Source: CAD feature listing. Evaluate the final solid. Frame: model axes, mm. Face numbers are marked on the shaded views. A direction names the side the tool comes from. Coordinates: 2 decimals unless noted, no trailing zeros. Order: outer loops, then holes, each group sorted by start corner. A loop starts at its lowest first (then second) coordinate and runs counter-clockwise, first axis right, second up.
Item 1: Contact query for flat-ended pins moving along their axis: P1, Ø0.8, axis at x = 2, z = 0, coming from the +Y side; P2, Ø2, axis at y = 1, z = -26, coming from the +X side; P3, Ø1.5, axis at y = 5, z = 0, coming from the -X side. Output: stop coordinate, or through.
Item 2: Section C-C on y = 5. Return the cut outline in (x, z), then the cut area to 3 significant figures.
Item 3: Reachability of the marked faces 1 and 2 from +Z, -Z, +X, -X, +Y, -Y: full face, straight path, thin tool, end or side. Return the list, or none.
Item 4: Section D-D on x = -3.25. Return the cut outline in (y, z), then the cut area to 3 significant figures.
Item 5: Section A-A on z = 0. Return the cut outline in (x, y).
Item 6: Ray query, line 1 (X direction, y = 6.85, z = 0); line 2 (Y direction, x = 1.75, z = -10). Return the intervals inside material, ascending.
Item 7: Section B-B on x = 1. Return the cut outline in (y, z).
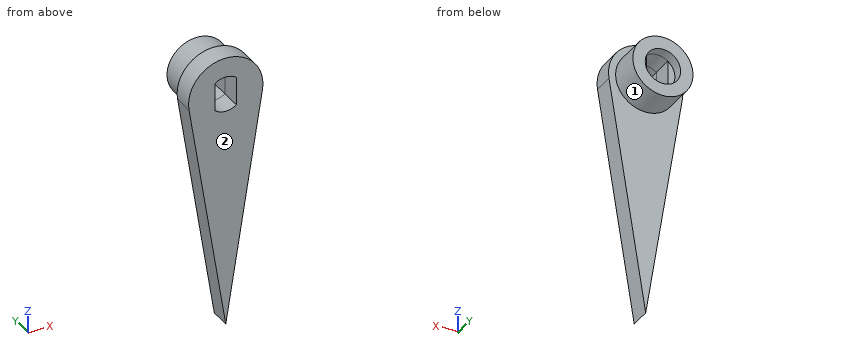
from build123d import *

# Parameters (mm, degrees)
SKETCH5_R           = 4.25
BOSS_EXTRUDE3_DEPTH = 7.5
SKETCH7_R           = 2.5
CUT_EXTRUDE2_DEPTH  = 1.5
CUT_EXTRUDE3_DEPTH  = 6
SKETCH9_R           = 5.25
BOSS_EXTRUDE4_DEPTH = 3


with BuildPart() as part:
    # Sketch5 → Boss-Extrude3 (new body)
    with BuildSketch(Plane(origin=(0, 0, 0), x_dir=(1, 0, 0), z_dir=(0, 1, 0))):
        Circle(SKETCH5_R)
    extrude(amount=BOSS_EXTRUDE3_DEPTH)

    # Sketch7 → Cut-Extrude2 (cut)
    with BuildSketch(Plane(origin=(0, 7.5, 0), x_dir=(1, 0, 0), z_dir=(0, 1, 0))):
        Circle(SKETCH7_R)
    extrude(amount=-CUT_EXTRUDE2_DEPTH, mode=Mode.SUBTRACT)

    # Sketch8 → Cut-Extrude3 (cut)
    with BuildSketch(Plane(origin=(0, 6, 0), x_dir=(1, 0, 0), z_dir=(0, 1, 0))):
        with BuildLine():
            Line((-1.5, -2), (-1.5, 2))
            ThreePointArc((-1.5, 2), (0, 2.5), (1.5, 2))
            Line((1.5, 2), (1.5, -2))
            ThreePointArc((1.5, -2), (0, -2.5), (-1.5, -2))
        make_face()
    extrude(amount=-CUT_EXTRUDE3_DEPTH, mode=Mode.SUBTRACT)

    # Sketch9 → Boss-Extrude4 (add)
    with BuildSketch(Plane(origin=(0, 0, 0), x_dir=(1, 0, 0), z_dir=(0, 1, 0))):
        with BuildLine():
            Line((0, 33.5), (-5.185129123, 0.822761194))
            ThreePointArc((-5.185129123, 0.822761194), (0, 5.25), (5.185129123, 0.822761194))
            Line((5.185129123, 0.822761194), (0, 33.5))
        make_face()
        Circle(SKETCH9_R)
        with BuildLine():
            ThreePointArc((1.5, 2), (0, 2.5), (-1.5, 2))
            Line((-1.5, 2), (-1.5, -2))
            ThreePointArc((-1.5, -2), (0, -2.5), (1.5, -2))
            Line((1.5, -2), (1.5, 2))
        make_face(mode=Mode.SUBTRACT)
    extrude(amount=BOSS_EXTRUDE4_DEPTH)


solid = part.part
Answer list:
1. P1: stops at y = 6
1. P2: stops at x = 1.35
1. P3: stops at x = -4.25
2. outline: circle Ø8.5 at (0, 0); hole (-1.5, -2) arc R2.5 ccw to (1.5, -2) - (1.5, 2) arc R2.5 ccw to (-1.5, 2) - close
2. area: 42.7 mm2
3. face 1: +Y
3. face 2: +Z, -Z, +X, -X, -Y
4. outline: (0, -13.02) - (3, -13.02) - (3, -2.74) - (7.5, -2.74) - (7.5, 2.74) - (3, 2.74) - (3, 4.12) - (0, 4.12) - close
4. area: 76.1 mm2
5. outline: (-5.25, 0) - (-1.5, 0) - (-1.5, 6) - (-2.5, 6) - (-2.5, 7.5) - (-4.25, 7.5) - (-4.25, 3) - (-5.25, 3) - close; (1.5, 0) - (5.25, 0) - (5.25, 3) - (4.25, 3) - (4.25, 7.5) - (2.5, 7.5) - (2.5, 6) - (1.5, 6) - close
6. line 1: x = -4.25 to -2.5, 2.5 to 4.25
6. line 2: y = 0 to 3
7. outline: (0, -27.2) - (3, -27.2) - (3, -4.13) - (7.5, -4.13) - (7.5, -2.29) - (0, -2.29) - close; (0, 2.29) - (7.5, 2.29) - (7.5, 4.13) - (3, 4.13) - (3, 5.15) - (0, 5.15) - close
